from build123d import *

# Parameters (mm, degrees)
ESQUISSE1_R             = 30
ESQUISSE1_R_2           = 19
BOSS_EXTRU_2_DEPTH      = 20
ESQUISSE5_R             = 2.55
ENL_V_MAT_EXTRU_3_DEPTH = 21
ESQUISSE6_R             = 4.2
ENL_V_MAT_EXTRU_4_DEPTH = 5.2


with BuildPart() as part:
    # Esquisse1 → Boss.-Extru.2 (new body)
    with BuildSketch(Plane(origin=(0, 0, 0), x_dir=(1, 0, 0), z_dir=(0, 1, 0))):
        Circle(ESQUISSE1_R)
        Circle(ESQUISSE1_R_2, mode=Mode.SUBTRACT)
    extrude(amount=BOSS_EXTRU_2_DEPTH)

    # Esquisse5 → Enlèv. mat.-Extru.3 (cut, through all)
    with BuildSketch(Plane(origin=(0, 20, 0), x_dir=(1, 0, 0), z_dir=(0, 1, 0))):
        with Locations((24.5, 0)):
            Circle(ESQUISSE5_R)
        with Locations((17.324116139, -17.324116139)):
            Circle(ESQUISSE5_R)
        with Locations((0, -24.5)):
            Circle(ESQUISSE5_R)
        with Locations((-17.324116139, -17.324116139)):
            Circle(ESQUISSE5_R)
        with Locations((-24.5, 0)):
            Circle(ESQUISSE5_R)
        with Locations((-17.324116139, 17.324116139)):
            Circle(ESQUISSE5_R)
        with Locations((0, 24.5)):
            Circle(ESQUISSE5_R)
        with Locations((17.324116139, 17.324116139)):
            Circle(ESQUISSE5_R)
    extrude(amount=-ENL_V_MAT_EXTRU_3_DEPTH, mode=Mode.SUBTRACT)

    # Esquisse6 → Enlèv. mat.-Extru.4 (cut)
    with BuildSketch(Plane(origin=(0, 20, 0), x_dir=(1, 0, 0), z_dir=(0, 1, 0))):
        with Locations((24.5, 0)):
            Circle(ESQUISSE6_R)
        with Locations((17.324116139, 17.324116139)):
            Circle(ESQUISSE6_R)
        with Locations((0, 24.5)):
            Circle(ESQUISSE6_R)
        with Locations((-17.324116139, 17.324116139)):
            Circle(ESQUISSE6_R)
        with Locations((-24.5, 0)):
            Circle(ESQUISSE6_R)
        with Locations((-17.324116139, -17.324116139)):
            Circle(ESQUISSE6_R)
        with Locations((0, -24.5)):
            Circle(ESQUISSE6_R)
        with Locations((17.324116139, -17.324116139)):
            Circle(ESQUISSE6_R)
    extrude(amount=-ENL_V_MAT_EXTRU_4_DEPTH, mode=Mode.SUBTRACT)


solid = part.part
CAD build for the part. Positions are in the model's coordinates, mm. A direction names the side the tool comes from. Round coordinates to 2 decimals unless told otherwise and drop trailing zeros. Write each loop counter-clockwise with the first axis right and the second up, starting at its lowest first coordinate (ties: lowest second). Pieces come first, ordered by that corner, then holes. Notation, with made-up numbers: M 4.5,-30 L 47.5,-30 A19 cw 47.5,1 Z; hole C 85.5,58.25 d1. An arc over 180 degrees is marked long. Put each result on its own line as item: value. Start each with the question number.
1) Saw through at D-D, the plane y = 6.75. Count the separate pieces of the cut face and the enclosed holes in it, and give its area (3 significant figures).
2) Saw through at B-B, the plane z = 0. Write the cut outline in (x, y), and give its area (3 significant figures).
3) Saw through at A-A, the plane x = 0. Write the cut outline in (y, z).
4) Pin check, flat tips, straight feed: pin 1 Ø1.5 at (y, z) = (5.5, 2) entering from -X; pin 2 Ø3 at (y, z) = (14, 22) entering from +X; pin 3 Ø8 at (x, z) = (0, -24.5) entering from -Y; pin 4 Ø6.5 at (x, z) = (0, -24.5) entering from +Y. Stop position of each tip, or through.
5) Saw through at C-C, the plane z = -11. Write the cut outline in (x, y), and give its area (3 significant figures).
6) Pull direction Z, two halves, no side cores. Call faces 3 (the cylindrical face through (-27.048, 7.504, -0.112)), 4 (the cylindrical face through (-15.95, 7.5, -19.47)), 5 (the flat face through (-14, 0, -14)): pulls with the +Z half, pulls with the -Z half, needs draft (parallel to the pull), parting line crosses it, or undercut.
7) 3-axis set-ups, long thin cutter, end or side, ignore diameter. For faces 1 (the cylindrical face through (-13.32, 17.44, -18.59)), 2 (the cylindrical face through (21.952, 7.504, -0.112)): which of +Z, -Z, +X, -X, +Y, -Y reach the whole face in a straight line?
8) Drill centre lines: probe 1 along Z at (x, y) = (0, 11.75); probe 2 along X at (y, z) = (17.3, 0). Where is each one in solid material? Low to high. Write a range as [from, to].
Resolved:
1. separate pieces: 1
1. enclosed holes: 9
1. area: 1,530 mm²
2. outline: M -30,0 L -27.05,0 L -27.05,14.8 L -28.7,14.8 L -28.7,20 L -30,20 Z; M -21.95,0 L -19,0 L -19,20 L -20.3,20 L -20.3,14.8 L -21.95,14.8 Z; M 19,0 L 21.95,0 L 21.95,14.8 L 20.3,14.8 L 20.3,20 L 19,20 Z; M 27.05,0 L 30,0 L 30,20 L 28.7,20 L 28.7,14.8 L 27.05,14.8 Z
2. area: 202 mm²
3. outline: M 0,-30 L 20,-30 L 20,-28.7 L 14.8,-28.7 L 14.8,-27.05 L 0,-27.05 Z; M 0,-21.95 L 14.8,-21.95 L 14.8,-20.3 L 20,-20.3 L 20,-19 L 0,-19 Z; M 0,19 L 20,19 L 20,20.3 L 14.8,20.3 L 14.8,21.95 L 0,21.95 Z; M 0,27.05 L 14.8,27.05 L 14.8,28.7 L 20,28.7 L 20,30 L 0,30 Z
4. pin 1: x = -29.97
4. pin 2: x = 21.9
4. pin 3: y = 0
4. pin 4: y = 14.8
5. outline: M -27.91,0 L -15.49,0 L -15.49,20 L -27.91,20 Z; M 15.49,0 L 27.91,0 L 27.91,20 L 15.49,20 Z
5. area: 497 mm²
6. face 3: undercut
6. face 4: undercut
6. face 5: needs draft
7. face 1: +Y
7. face 2: +Y, -Y
8. probe 1: [-30, -27.05], [-21.95, -19], [19, 21.95], [27.05, 30]
8. probe 2: [-30, -28.7], [-20.3, -19], [19, 20.3], [28.7, 30]
